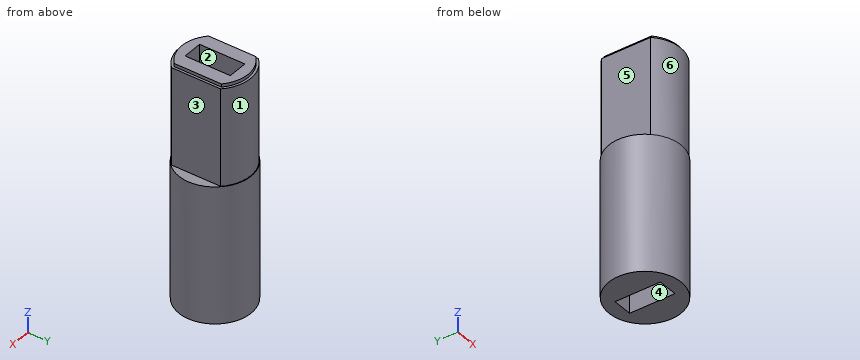
from build123d import *

# Parameters (mm, degrees)
SKETCH2_R           = 4.57
BOSS_EXTRUDE1_DEPTH = 17.3
BOSS_EXTRUDE3_DEPTH = 12.7
SKETCH5_W           = 2.5
SKETCH5_H           = 5.74
CUT_EXTRUDE1_DEPTH  = 31
SKETCH6_R           = 4.5
CUT_EXTRUDE3_DEPTH  = 0.4


with BuildPart() as part:
    # Sketch2 → Boss-Extrude1 (new body)
    with BuildSketch(Plane.XY):
        Circle(SKETCH2_R)
    extrude(amount=BOSS_EXTRUDE1_DEPTH)

    # Sketch4 → Boss-Extrude3 (add)
    with BuildSketch(Plane.XY.offset(17.3)):
        with BuildLine():
            Line((-3.25, 3.112474899), (-3.25, -3.112474899))
            ThreePointArc((-3.25, -3.112474899), (0, -4.5), (3.25, -3.112474899))
            Line((3.25, -3.112474899), (3.25, 3.112474899))
            ThreePointArc((3.25, 3.112474899), (0, 4.5), (-3.25, 3.112474899))
        make_face()
    extrude(amount=BOSS_EXTRUDE3_DEPTH)

    # Sketch5 → Cut-Extrude1 (cut, through all)
    with BuildSketch(Plane.XY.offset(30)):
        Rectangle(SKETCH5_W, SKETCH5_H)
    extrude(amount=-CUT_EXTRUDE1_DEPTH, mode=Mode.SUBTRACT)

    # Sketch6 → Cut-Extrude3 (cut)
    with BuildSketch(Plane.XY.offset(30)):
        Circle(SKETCH6_R)
        with BuildLine():
            Line((-2.95, 2.989565186), (-2.95, -2.989565186))
            ThreePointArc((-2.95, -2.989565186), (0, -4.2), (2.95, -2.989565186))
            Line((2.95, -2.989565186), (2.95, 2.989565186))
            ThreePointArc((2.95, 2.989565186), (0, 4.2), (-2.95, 2.989565186))
        make_face(mode=Mode.SUBTRACT)
    extrude(amount=-CUT_EXTRUDE3_DEPTH, mode=Mode.SUBTRACT)


solid = part.part
The model under review builds one solid part; all positions refer to its coordinate system, in mm. Face numbers are marked on the shaded views. A direction names the side the tool comes from. Round coordinates to 2 decimals unless told otherwise and drop trailing zeros. Loops run counter-clockwise (first coordinate to the right, second up) from the corner with the lowest first, then second, coordinate; pieces in that order, holes last. Notation, with made-up numbers: (-34, -36) -> (-28, -36) arc R26 cw to (-28, -9) -> close; hole circle Ø8 at (79, -19.75). An arc over 180 degrees is marked (long way). One line per question, with ' | ' between items. Start each with the question number.
Item 1: Draft analysis for pull direction X (two halves, no side actions). For the marked faces 4, 5 and 6, state which applies: +X half, -X half, draft (parallel to the pull), parting line (faces both ways), or undercut.
Item 2: Add section A-A, the plane x = 0. Write out the cut boundary in (y, z).
Item 3: Add section B-B, the plane z = 24.5. Write out the cut boundary in (x, y).
Item 4: Add section C-C, the plane y = 0. Write out the cut boundary in (x, z), then the cut area to 3 significant figures.
Item 5: For pin 1 (3 mm diameter, centred on x = -0.5, z = 11, fed in from -Y); pin 2 (1.5 mm diameter, centred on y = 2, z = 27, fed in from -X); pin 3 (3 mm diameter, centred on y = -1.5, z = 20.5, fed in from +X); pin 4 (2 mm diameter, centred on x = 2.5, z = 13.5, fed in from +Y), all flat-tipped, find the tip position at first contact; note any pin that passes through.
Item 6: Wall thickness on line 1 along X through (y, z) = (-0.5, 19); line 2 along Y through (x, z) = (-0.25, 22); line 3 along X through (y, z) = (-0.25, 11.25): over which ranges is each line inside the solid? List them lowest first. Write a range as [from, to].
Item 7: Add section D-D, the plane z = 4.5. Write out the cut boundary in (x, y).
Item 8: Machinability: for the marked faces 1, 2 and 3, which of the approach directions +Z, -Z, +X, -X, +Y, -Y give a long, thin tool a straight path to every point of the face, cutting with its end or side? Answer none if there is none.
Return value:
1) face 4: undercut | face 5: -X half | face 6: parting line
2) outline: (-4.57, 0) -> (-2.87, 0) -> (-2.87, 30) -> (-4.2, 30) -> (-4.2, 29.6) -> (-4.5, 29.6) -> (-4.5, 17.3) -> (-4.57, 17.3) -> close; (2.87, 0) -> (4.57, 0) -> (4.57, 17.3) -> (4.5, 17.3) -> (4.5, 29.6) -> (4.2, 29.6) -> (4.2, 30) -> (2.87, 30) -> close
3) outline: (-3.25, -3.11) arc R4.5 ccw to (3.25, -3.11) -> (3.25, 3.11) arc R4.5 ccw to (-3.25, 3.11) -> close; hole (-1.25, -2.87) -> (1.25, -2.87) -> (1.25, 2.87) -> (-1.25, 2.87) -> close
4) outline: (-4.57, 0) -> (-1.25, 0) -> (-1.25, 30) -> (-2.95, 30) -> (-2.95, 29.6) -> (-3.25, 29.6) -> (-3.25, 17.3) -> (-4.57, 17.3) -> close; (1.25, 0) -> (4.57, 0) -> (4.57, 17.3) -> (3.25, 17.3) -> (3.25, 29.6) -> (2.95, 29.6) -> (2.95, 30) -> (1.25, 30) -> close | area: 165 mm2
5) pin 1: stops at y = -4.57 | pin 2: stops at x = -3.25 | pin 3: stops at x = 3.25 | pin 4: stops at y = 4.32
6) line 1: x = [-3.25, -1.25], [1.25, 3.25] | line 2: y = [-4.49, -2.87], [2.87, 4.49] | line 3: x = [-4.56, -1.25], [1.25, 4.56]
7) outline: circle Ø9.14 at (0, 0); hole (-1.25, -2.87) -> (1.25, -2.87) -> (1.25, 2.87) -> (-1.25, 2.87) -> close
8) face 1: +Z, +Y | face 2: +Z, -Z | face 3: +Z, +X, +Y, -Y
